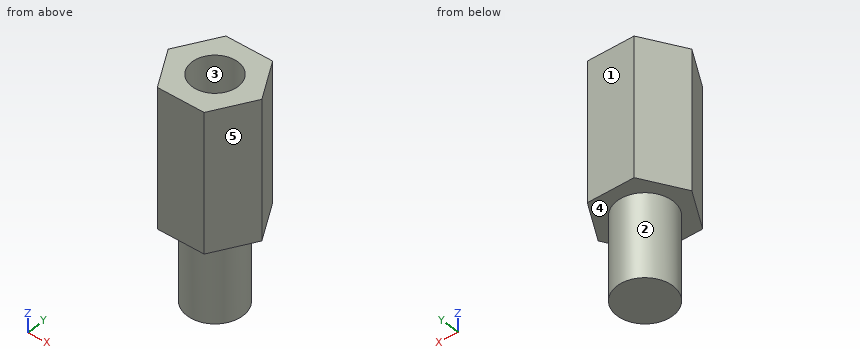
```python
from build123d import *

# Parameters (mm, degrees)
EXTRUDE_1_DEPTH     = 10
SKETCH_2_R          = 2
EXTRUDE_2_DEPTH     = 6
SKETCH_3_R          = 1.65
CUT_EXTRUDE_1_DEPTH = 5


with BuildPart() as part:
    # 草圖1 → 填料-伸長1 (new body)
    with BuildSketch(Plane.XY):
        Polygon((1.675, 2.901185103), (-1.675, 2.901185103), (-3.35, 0), (-1.675, -2.901185103), (1.675, -2.901185103), (3.35, 0), align=None)
    extrude(amount=EXTRUDE_1_DEPTH)

    # 草圖2 → 填料-伸長2 (add)
    with BuildSketch(Plane(origin=(0, 0, 0), x_dir=(-1, 0, 0), z_dir=(0, 0, -1))):
        Circle(SKETCH_2_R)
    extrude(amount=EXTRUDE_2_DEPTH)

    # 草圖3 → 除料-伸長1 (cut)
    with BuildSketch(Plane.XY.offset(10)):
        Circle(SKETCH_3_R)
    extrude(amount=-CUT_EXTRUDE_1_DEPTH, mode=Mode.SUBTRACT)


solid = part.part
```
Build history of the part. All positions in model axes, mm. Face numbers are marked on the shaded views. A direction names the side the tool comes from. Coordinates: 2 decimals unless noted, no trailing zeros. Order: outer loops, then holes, each group sorted by start corner. A loop starts at its lowest first (then second) coordinate and runs counter-clockwise, first axis right, second up. Notation, with made-up numbers: (6.5, 36.25) -> (31.5, 36.25) arc R8 ccw to (31.5, 41.25) -> close; hole circle Ø9 at (37.25, -10.75). An arc over 180 degrees is marked (long way). Answer in a Markdown table with one row per item. Add a question column.
Q1. Band-saw the part on C-C, the plane y = 0.6. List the corners of the cut face in (x, z).
Q2. Wall check: line 1 along Y through (x, z) = (0, 8.55); line 2 along Z through (x, y) = (-1, 2.35); line 3 along Y through (x, z) = (-1, 8.5). Give the ranges that are in metal, low to high. Write a range as [from, to].
Q3. Drop a flat-ended pin along its axis: pin 1 (3 mm diameter, centred on y = 2, z = 3.5, fed in from +X). Give the stop position or say it passes through.
Q4. Band-saw the part on B-B, the plane x = 0. List the corners of the cut face in (y, z), then the cut area to 3 significant figures.
Q5. Band-saw the part on A-A, the plane z = 7. List the corners of the cut face in (x, y) (3 decimals).
Q6. Band-saw the part on D-D, the plane z = 3.5. List the corners of the cut face in (x, y) (3 decimals).
Q7. Mould opens along X. For the marked faces 3, 4 and 5 say: +X half, -X half, draft (parallel to the pull), parting line (faces both ways), or undercut.
Q8. Which spindle directions (+Z, -Z, +X, -X, +Y, -Y) get a long thin tool onto all of the face, cutting with end or side? Do the marked faces 1 and 2. Say none if no direction does.
Answers follow:
| question | item | result |
|---|---|---|
| 1 | outline | (-3, 0) -> (-1.91, 0) -> (-1.91, -6) -> (1.91, -6) -> (1.91, 0) -> (3, 0) -> (3, 10) -> (1.54, 10) -> (1.54, 5) -> (-1.54, 5) -> (-1.54, 10) -> (-3, 10) -> close |
| 2 | line 1 | [-2.9, -1.65], [1.65, 2.9] |
| 2 | line 2 | [0, 10] |
| 2 | line 3 | [-2.9, -1.31], [1.31, 2.9] |
| 3 | pin 1 | x = 3.06 |
| 4 | outline | (-2.9, 0) -> (-2, 0) -> (-2, -6) -> (2, -6) -> (2, 0) -> (2.9, 0) -> (2.9, 10) -> (1.65, 10) -> (1.65, 5) -> (-1.65, 5) -> (-1.65, 10) -> (-2.9, 10) -> close |
| 4 | area | 65.5 mm^2 |
| 5 | outline | (-3.35, 0) -> (-1.675, -2.901) -> (1.675, -2.901) -> (3.35, 0) -> (1.675, 2.901) -> (-1.675, 2.901) -> close; hole circle Ø3.3 at (0, 0) |
| 6 | outline | (-3.35, 0) -> (-1.675, -2.901) -> (1.675, -2.901) -> (3.35, 0) -> (1.675, 2.901) -> (-1.675, 2.901) -> close |
| 7 | face 3 | undercut |
| 7 | face 4 | draft |
| 7 | face 5 | +X half |
| 8 | face 1 | +Z, -Z, +X, -X, +Y |
| 8 | face 2 | -Z |
